Work out the finished part from the listing and answer in its coordinate system (mm). A direction names the side the tool comes from. Round coordinates to 2 decimals unless told otherwise and drop trailing zeros. Write each loop counter-clockwise with the first axis right and the second up, starting at its lowest first coordinate (ties: lowest second). Pieces come first, ordered by that corner, then holes. Notation, with made-up numbers: M 47,-34 L 68,-34 A19 ccw 68,-24 Z; hole C 63,67.5 d4. An arc over 180 degrees is marked long. Answer in a Markdown table with one row per item.
Autodesk Fusion 360 part; units mm, degrees
sketch "baseplate" plane through (0, 0, 0) normal (0, 1, 0) x (1, 0, 0)
  line L0 (0, 0) -> (80, 0)
  line L1 (80, 0) -> (80, -40)
  line L2 (80, -40) -> (0, -40)
  line L3 (0, -40) -> (0, 0)
  dimension "d1" = 80
  dimension "d2" = 40
sketch "pryamid_base" plane through (0, 0, 0) normal (0, 1, 0) x (1, 0, 0)
  line L0 (5, -35) -> (15, -35)
  line L1 (15, -35) -> (15, -25)
  line L2 (15, -25) -> (5, -25)
  line L3 (5, -25) -> (5, -35)
  line L4 (35, -35) -> (35, -25)
  line L5 (35, -25) -> (25, -25)
  line L6 (25, -35) -> (35, -35)
  line L7 (25, -25) -> (25, -35)
  line L8 (75, -35) -> (75, -25)
  line L9 (45, -35) -> (55, -35)
  line L10 (55, -25) -> (45, -25)
  line L11 (65, -25) -> (65, -35)
  line L12 (65, -35) -> (75, -35)
  line L13 (55, -35) -> (55, -25)
  line L14 (45, -25) -> (45, -35)
  line L15 (75, -25) -> (65, -25)
  line L16 (35, -5) -> (25, -5)
  line L17 (35, -15) -> (35, -5)
  line L18 (15, -5) -> (5, -5)
  line L19 (25, -5) -> (25, -15)
  line L20 (45, -15) -> (55, -15)
  line L21 (55, -15) -> (55, -5)
  line L22 (5, -5) -> (5, -15)
  line L23 (45, -5) -> (45, -15)
  line L24 (75, -15) -> (75, -5)
  line L25 (65, -5) -> (65, -15)
  line L26 (75, -5) -> (65, -5)
  line L27 (55, -5) -> (45, -5)
  line L28 (65, -15) -> (75, -15)
  line L29 (5, -15) -> (15, -15)
  line L30 (15, -15) -> (15, -5)
  line L31 (25, -15) -> (35, -15)
  dimension "d3" = 10
  dimension "d4" = 10
  dimension "d5" = 10
  dimension "d6" = 10
  dimension "d7" = 10
  dimension "d8" = 10
  dimension "d9" = 10
  dimension "d10" = 10
  dimension "d11" = 10
  dimension "d12" = 10
  dimension "d13" = 10
  dimension "d14" = 10
  dimension "d15" = 10
  dimension "d16" = 10
  dimension "d17" = 10
  dimension "d18" = 10
ref_plane "WorkPlane1" through (0, 4.5, 0) normal (0, 1, 0) x (0, 0, 1)
sketch "pryamid_offsetplane" plane through (0, 4.5, 0) normal (0, 1, 0) x (1, 0, 0)
  line L0 (7.5, -32.5) -> (12.5, -32.5)
  line L1 (12.5, -32.5) -> (12.5, -27.5)
  line L2 (12.5, -27.5) -> (7.5, -27.5)
  line L3 (7.5, -27.5) -> (7.5, -32.5)
  line L4 (27.5, -27.5) -> (27.5, -32.5)
  line L5 (32.5, -32.5) -> (32.5, -27.5)
  line L6 (27.5, -32.5) -> (32.5, -32.5)
  line L7 (32.5, -27.5) -> (27.5, -27.5)
  line L8 (7.5, -27.5) -> (7.5, -32.5)
  line L9 (12.5, -32.5) -> (12.5, -27.5)
  line L10 (7.5, -32.5) -> (12.5, -32.5)
  line L11 (12.5, -27.5) -> (7.5, -27.5)
  line L12 (47.5, -27.5) -> (47.5, -32.5)
  line L13 (52.5, -32.5) -> (52.5, -27.5)
  line L14 (47.5, -32.5) -> (52.5, -32.5)
  line L15 (52.5, -27.5) -> (47.5, -27.5)
  line L16 (67.5, -27.5) -> (67.5, -32.5)
  line L17 (72.5, -32.5) -> (72.5, -27.5)
  line L18 (67.5, -32.5) -> (72.5, -32.5)
  line L19 (72.5, -27.5) -> (67.5, -27.5)
  line L20 (72.5, -12.5) -> (72.5, -7.5)
  line L21 (27.5, -7.5) -> (27.5, -12.5)
  line L22 (12.5, -12.5) -> (12.5, -7.5)
  line L23 (72.5, -7.5) -> (67.5, -7.5)
  line L24 (12.5, -7.5) -> (7.5, -7.5)
  line L25 (52.5, -12.5) -> (52.5, -7.5)
  line L26 (7.5, -7.5) -> (7.5, -12.5)
  line L27 (7.5, -12.5) -> (12.5, -12.5)
  line L28 (47.5, -12.5) -> (52.5, -12.5)
  line L29 (67.5, -7.5) -> (67.5, -12.5)
  line L30 (47.5, -7.5) -> (47.5, -12.5)
  line L31 (67.5, -12.5) -> (72.5, -12.5)
  line L32 (32.5, -7.5) -> (27.5, -7.5)
  line L33 (52.5, -7.5) -> (47.5, -7.5)
  line L34 (27.5, -12.5) -> (32.5, -12.5)
  line L35 (12.5, -7.5) -> (7.5, -7.5)
  line L36 (32.5, -12.5) -> (32.5, -7.5)
  line L37 (12.5, -12.5) -> (12.5, -7.5)
  line L38 (7.5, -12.5) -> (12.5, -12.5)
  line L39 (7.5, -7.5) -> (7.5, -12.5)
extrude "Extrude1" add sketch "baseplate" against normal blind 5
loft "Loft1" add profiles "pryamid_base", "pryamid_offsetplane" section 1 contours L0 L1 L2 L3 section 2 contours L0 L1 L2 L3 L8 L9 L10 L11
loft "Loft2" add profiles "pryamid_base", "pryamid_offsetplane" section 1 contours L4 L5 L6 L7 section 2 contours L4 L5 L6 L7
loft "Loft3" add profiles "pryamid_base", "pryamid_offsetplane" section 1 contours L9 L10 L13 L14 section 2 contours L12 L13 L14 L15
loft "Loft4" add profiles "pryamid_base", "pryamid_offsetplane" section 1 contours L8 L11 L12 L15 section 2 contours L16 L17 L18 L19
loft "Loft5" add profiles "pryamid_base", "pryamid_offsetplane" section 1 contours L24 L25 L26 L28 section 2 contours L20 L23 L29 L31
loft "Loft6" add profiles "pryamid_base", "pryamid_offsetplane" section 1 contours L20 L21 L23 L27 section 2 contours L25 L28 L30 L33
loft "Loft7" add profiles "pryamid_base", "pryamid_offsetplane" section 1 contours L16 L17 L19 L31 section 2 contours L21 L32 L34 L36
loft "Loft8" add profiles "pryamid_base", "pryamid_offsetplane" section 1 contours L18 L22 L29 L30 section 2 contours L22 L24 L26 L27 L35 L37 L38 L39
sketch "sidewall" plane through (0, 0, 0) normal (0, 1, 0) x (1, 0, 0)
  line L0 (0, 0) -> (-8, 0)
  line L1 (-8, 0) -> (-8, -40)
  line L2 (-8, -40) -> (0, -40)
  line L3 (0, -40) -> (0, 0)
  dimension "d22" = 8
extrude "Extrude2" add sketch "sidewall" along normal blind 40 and the other way blind 5
sketch "sidemount" plane through (0, 0, 0) normal (0, 1, 0) x (1, 0, 0)
  line L0 (80, 0) -> (88, 0)
  line L1 (88, 0) -> (88, -40)
  line L2 (88, -40) -> (80, -40)
  line L3 (80, -40) -> (80, 0)
extrude "Extrude3" add sketch "sidemount" against normal blind 5
sketch "holes" plane through (0, -5, 0) normal (0, -1, 0) x (1, 0, 0)
  line L0 (88, 40) -> (-8, 40)
  line L1 (-8, 40) -> (-8, 0)
  line L2 (-8, 0) -> (88, 0)
  line L3 (88, 0) -> (88, 40)
  line L4 (-8, 0) -> (-4, 0)
  line L5 (-8, 6) -> (-8, 0)
  line L6 (-4, 40) -> (-8, 40)
  line L7 (-8, 40) -> (-8, 34)
  circle A0 centre (-4, 34) radius 2
  circle A1 centre (-4, 6) radius 2
  circle A2 centre (-4, 34) radius 3.4
  circle A3 centre (-4, 6) radius 3.4
  dimension "d29" = 6
  dimension "d30" = 4
  dimension "d31" = 4
  dimension "d32" = 6.8
  dimension "d33" = 6.8
extrude "Extrude4" cut sketch "holes" against normal blind 51 contours A0 | A1
extrude "Extrude5" cut sketch "holes" against normal blind 5 contours A2 | A3
sketch "Sketch7" plane through (0, -5, 0) normal (0, -1, 0) x (1, 0, 0)
  circle A0 centre (84, 34) radius 2
  circle A1 centre (84, 6) radius 2
  circle A2 centre (84, 34) radius 3.4
  circle A3 centre (84, 6) radius 3.4
  dimension "d42" = 4
  dimension "d43" = 4
  dimension "d44" = 6.8
  dimension "d45" = 6.8
extrude "Extrude6" cut sketch "Sketch7" against normal blind 16 contours A0 | A1
1. Determine the mould class of faces 4 (the flat face through (88, -2, 20)), 5 (the flat face through (70, 4.5, 10)), 6 (the cylindrical face through (85.908, -2.535, 6.601)), 7 (the flat face through (43, 0, 20)) for opening direction X: released by +X, released by -X, zero draft, split by the parting line, or undercut.
Calculated:
| item | result |
|---|---|
| face 4 | released by +X |
| face 5 | zero draft |
| face 6 | undercut |
| face 7 | undercut |
2. Given pin 1 (1.5 mm diameter, centred on x = 11, z = 29.5, fed in from +Y); pin 2 (2.5 mm diameter, centred on x = 84, z = 6, fed in from -Y); pin 3 (4 mm diameter, centred on y = 23.5, z = 8.5, fed in from +X); pin 4 (9 mm diameter, centred on x = -4, z = 6, fed in from +Y), each flat-ended and moving along its own axis, determine where each tip first touches the part or whether it passes through.
Calculated:
| item | result |
|---|---|
| pin 1 | stops at y = 4.5 |
| pin 2 | passes through |
| pin 3 | stops at x = 0 |
| pin 4 | stops at y = 40 |
3. The part is cut by section B-B (y = 15). Determine the outline of the cut face in (x, z).
Calculated:
| item | result |
|---|---|
| outline | M -8,0 L 0,0 L 0,40 L -8,40 Z; hole C -4,6 d4; hole C -4,34 d4 |
4. A tool of negligible diameter and unlimited length cuts with its end or side. For faces 1 (the flat face through (70, 4.5, 30)), 2 (the flat face through (-4, 40, 20)), 3 (the cylindrical face through (-0.86, -2.54, 32.7)), from which of +Z, -Z, +X, -X, +Y, -Y can it reach the whole face along a straight path? Write none if from no direction.
Calculated:
| item | result |
|---|---|
| face 1 | +Z, -Z, +X, +Y |
| face 2 | +Z, -Z, +X, -X, +Y |
| face 3 | -Y |
5. The part is cut by section C-C (z = 34). Count the separate pieces of the cut face and the enclosed holes in it, plus the area to 3 significant figures.
Calculated:
| item | result |
|---|---|
| separate pieces | 3 |
| enclosed holes | 0 |
| area | 651 mm² |
6. The part is cut by section A-A (x = -4). Determine the outline of the cut face in (y, z), plus the area to 3 significant figures.
Calculated:
| item | result |
|---|---|
| outline | M -5,0 L 40,0 L 40,4 L 0,4 L 0,2.6 L -5,2.6 Z; M -5,9.4 L 0,9.4 L 0,8 L 40,8 L 40,32 L 0,32 L 0,30.6 L -5,30.6 Z; M -5,37.4 L 0,37.4 L 0,36 L 40,36 L 40,40 L -5,40 Z |
| area | 1,410 mm² |
7. Consider line 1 along Z through (x, y) = (-4, 24); line 2 along Y through (x, z) = (28, 9); line 3 along Y through (x, z) = (23.5, 2). Determine where each line is inside the solid, lowest interval first. Write a range as from..to.
Calculated:
| item | result |
|---|---|
| line 1 | z = 0..4, 8..32, 36..40 |
| line 2 | y = -5..4.5 |
| line 3 | y = -5..0 |
8. The part is cut by section D-D (x = 84). Determine the outline of the cut face in (y, z), plus the area to 3 significant figures.
Calculated:
| item | result |
|---|---|
| outline | M -5,0 L 0,0 L 0,4 L -5,4 Z; M -5,8 L 0,8 L 0,32 L -5,32 Z; M -5,36 L 0,36 L 0,40 L -5,40 Z |
| area | 160 mm² |
